CAD build for the part. Positions are in the model's coordinates, mm. Face numbers are marked on the shaded views. Coordinates: 2 decimals unless noted, no trailing zeros. Loops run counter-clockwise (first coordinate to the right, second up) from the corner with the lowest first, then second, coordinate; pieces in that order, holes last. Notation, with made-up numbers: (23.25, -9.5) -> (38.25, -9.5) arc R17 ccw to (38.25, 14.5) -> close; hole circle Ø10 at (18.25, 66). An arc over 180 degrees is marked (long way). Answer as a JSON object with one key per item and string values. Group by question number.
from build123d import *

# Parameters (mm, degrees)
SKETCH1_W           = 45
SKETCH1_H           = 25
BOSS_EXTRUDE1_DEPTH = 32
SKETCH2_R           = 11
BOSS_EXTRUDE2_DEPTH = 5
BOSS_EXTRUDE3_DEPTH = 2.5
SKETCH4_W           = 31
SKETCH4_H           = 5
BOSS_EXTRUDE4_DEPTH = 3
SKETCH5_W           = 31
SKETCH5_H           = 5
BOSS_EXTRUDE5_DEPTH = 3
SKETCH6_W           = 25
SKETCH6_H           = 5
BOSS_EXTRUDE6_DEPTH = 3


with BuildPart() as part:
    # Sketch1 → Boss-Extrude1 (new body)
    with BuildSketch(Plane(origin=(0, 0, 0), x_dir=(1, 0, 0), z_dir=(0, 1, 0))):
        Rectangle(SKETCH1_W, SKETCH1_H)
    extrude(amount=BOSS_EXTRUDE1_DEPTH)

    # Sketch2 → Boss-Extrude2 (add)
    with BuildSketch(Plane(origin=(0, 32, 0), x_dir=(1, 0, 0), z_dir=(0, 1, 0))):
        with Locations((-11.5, 0)):
            Circle(SKETCH2_R)
    extrude(amount=BOSS_EXTRUDE2_DEPTH)

    # Sketch3 → Boss-Extrude3 (add)
    with BuildSketch(Plane(origin=(0, 32, 0), x_dir=(1, 0, 0), z_dir=(0, 1, 0))):
        with BuildLine():
            Line((-4.952747944, 9.555141067), (20.5, 9.555141067))
            Line((20.5, 9.555141067), (20.5, -9.555141067))
            Line((20.5, -9.555141067), (-4.952747944, -9.555141067))
            ThreePointArc((-4.952747944, -9.555141067), (0.083057899, 0), (-4.952747944, 9.555141067))
        make_face()
    extrude(amount=BOSS_EXTRUDE3_DEPTH)

    # Sketch4 → Boss-Extrude4 (add)
    with BuildSketch(Plane.XY.offset(12.5)):
        with Locations((7, 29.5)):
            Rectangle(SKETCH4_W, SKETCH4_H)
        with Locations((7, 2.5)):
            Rectangle(SKETCH4_W, SKETCH4_H)
    extrude(amount=BOSS_EXTRUDE4_DEPTH)

    # Sketch5 → Boss-Extrude5 (add)
    with BuildSketch(Plane(origin=(0, 0, -12.5), x_dir=(-1, 0, 0), z_dir=(0, 0, -1))):
        with Locations((-7, 29.5)):
            Rectangle(SKETCH5_W, SKETCH5_H)
        with Locations((-7, 2.5)):
            Rectangle(SKETCH5_W, SKETCH5_H)
    extrude(amount=BOSS_EXTRUDE5_DEPTH)

    # Sketch6 → Boss-Extrude6 (add)
    with BuildSketch(Plane(origin=(22.5, 0, 0), x_dir=(0, 0, -1), z_dir=(1, 0, 0))):
        with Locations((0, 2.5)):
            Rectangle(SKETCH6_W, SKETCH6_H)
        with Locations((0, 29.5)):
            Rectangle(SKETCH6_W, SKETCH6_H)
    extrude(amount=BOSS_EXTRUDE6_DEPTH)


solid = part.part
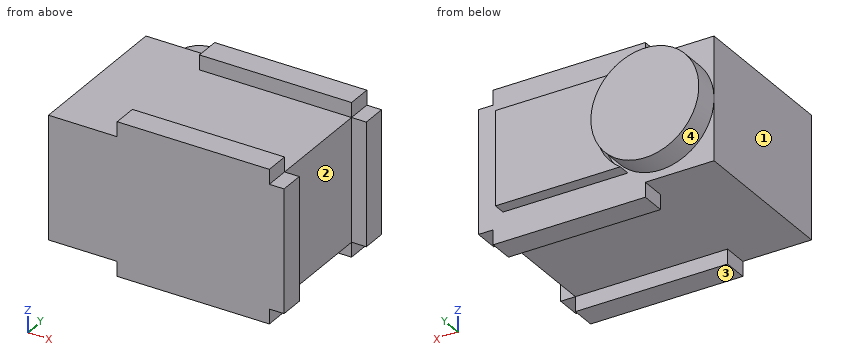
Item 1: Flat gauge pins, fed straight in: P1, Ø5.5, axis at x = 12.5, z = -3, coming from the +Y side; P2, Ø9.5, axis at x = -2, y = 21.5, coming from the -Z side; P3, Ø0.9, axis at y = 3.5, z = -14, coming from the +X side; P4, Ø1.5, axis at x = 24, z = -5, coming from the -Y side. Where does each tip first touch, or does it go through?
Item 2: Band-saw the part on A-A, the plane y = 33. List the corners of the cut face in (x, z), and give its area (3 significant figures).
Item 3: Band-saw the part on D-D, the plane z = -6.5. List the corners of the cut face in (x, y), and give its area (3 significant figures).
Item 4: Band-saw the part on C-C, the plane y = 3.5. List the corners of the cut face in (x, z).
Item 5: Band-saw the part on B-B, the plane x = 11. List the corners of the cut face in (y, z).
Item 6: Pull direction X, two halves, no side cores. Call the marked faces 1, 2, 3 and 4: +X half, -X half, draft (parallel to the pull), parting line (faces both ways), or undercut.
Item 7: Drill centre lines: L1, parallel to Y at x = 7, z = -13.5; L2, parallel to X at y = 8.5, z = 8; L3, parallel to Z at x = -9, y = 9. Where is each one in solid material? Low to high.
Reply:
{
 "1": {"P1": "y = 34.5", "P2": "z = -12.5", "P3": "x = 22.5", "P4": "y = 0"},
 "2": {"outline": "circle Ø22 at (-11.5, 0); (-4.95, -9.56) -> (20.5, -9.56) -> (20.5, 9.56) -> (-4.95, 9.56) arc R11.58 cw to start", "area": "799 mm²"},
 "3": {"outline": "(-22.5, 0) -> (25.5, 0) -> (25.5, 5) -> (22.5, 5) -> (22.5, 27) -> (25.5, 27) -> (25.5, 32) -> (20.5, 32) -> (20.5, 34.5) -> (-1.91, 34.5) -> (-1.91, 32) -> (-2.63, 32) -> (-2.63, 37) -> (-20.37, 37) -> (-20.37, 32) -> (-22.5, 32) -> close", "area": "1,610 mm²"},
 "4": {"outline": "(-22.5, -12.5) -> (-8.5, -12.5) -> (-8.5, -15.5) -> (22.5, -15.5) -> (22.5, -12.5) -> (25.5, -12.5) -> (25.5, 12.5) -> (22.5, 12.5) -> (22.5, 15.5) -> (-8.5, 15.5) -> (-8.5, 12.5) -> (-22.5, 12.5) -> close"},
 "5": {"outline": "(0, -15.5) -> (5, -15.5) -> (5, -12.5) -> (27, -12.5) -> (27, -15.5) -> (32, -15.5) -> (32, -9.56) -> (34.5, -9.56) -> (34.5, 9.56) -> (32, 9.56) -> (32, 15.5) -> (27, 15.5) -> (27, 12.5) -> (5, 12.5) -> (5, 15.5) -> (0, 15.5) -> close"},
 "6": {"face 1": "-X half", "face 2": "+X half", "face 3": "draft", "face 4": "undercut"},
 "7": {"L1": "0 to 5, 27 to 32", "L2": "-22.5 to 22.5", "L3": "-12.5 to 12.5"}
}
